Can you work these out from the drawing? Everything is in mm from the part's minimum corner. A direction names the side the tool comes from. Give positions to 0.01 mm unless a question says otherwise; leave off trailing zeros. Order: outer loops, then holes, each group sorted by start corner. A loop starts at its lowest first (then second) coordinate and runs counter-clockwise, first axis right, second up. Notation, with made-up numbers: (76.5, -9.75) -> (86.5, -9.75) arc R15 cw to (86.5, 15.25) -> close; hole circle Ø6 at (53.25, 24.5). An arc over 180 degrees is marked (long way). Answer as CSV lines item,"result". Start each with the question number.
(1) I want a section at B-B (z = 7.5). Please give me the cut outline in (x, y) (3 decimals), plus the area to 4 significant figures.
(2) I need wall thicknesses on L1, parallel to Y at x = 16.5, z = 5.25; L2, parallel to X at y = 7, z = 5.25; L3, parallel to X at y = 5.25, z = 8.5. Which ranges of each line are inside material? Lowest first, please.
(3) On a 3-axis mill with a long thin cutter (end or side, diameter ignored), from which of +Z, -Z, +X, -X, +Y, -Y can I reach the whole of each face in a straight line? I mean the marked faces 1 and 2. Say none if no direction works.
(4) I want a section at C-C (y = 5). Please give me the cut outline in (x, z) (3 decimals), plus the area to 3 significant figures.
(5) I want a section at A-A (x = 29.09). Please give me the cut outline in (y, z) (3 decimals).
(6) Will these pins go through, and if not, where does the flat tip stop? pin 1 Ø6 at (x, y) = (30, 7) entering from +Z (3 decimals); pin 2 Ø7.5 at (x, z) = (16.5, 10) entering from +Y; pin 3 Ø1 at (x, y) = (30.5, 9.5) entering from -Z.
(7) I want a section at D-D (x = 10). Please give me the cut outline in (y, z).
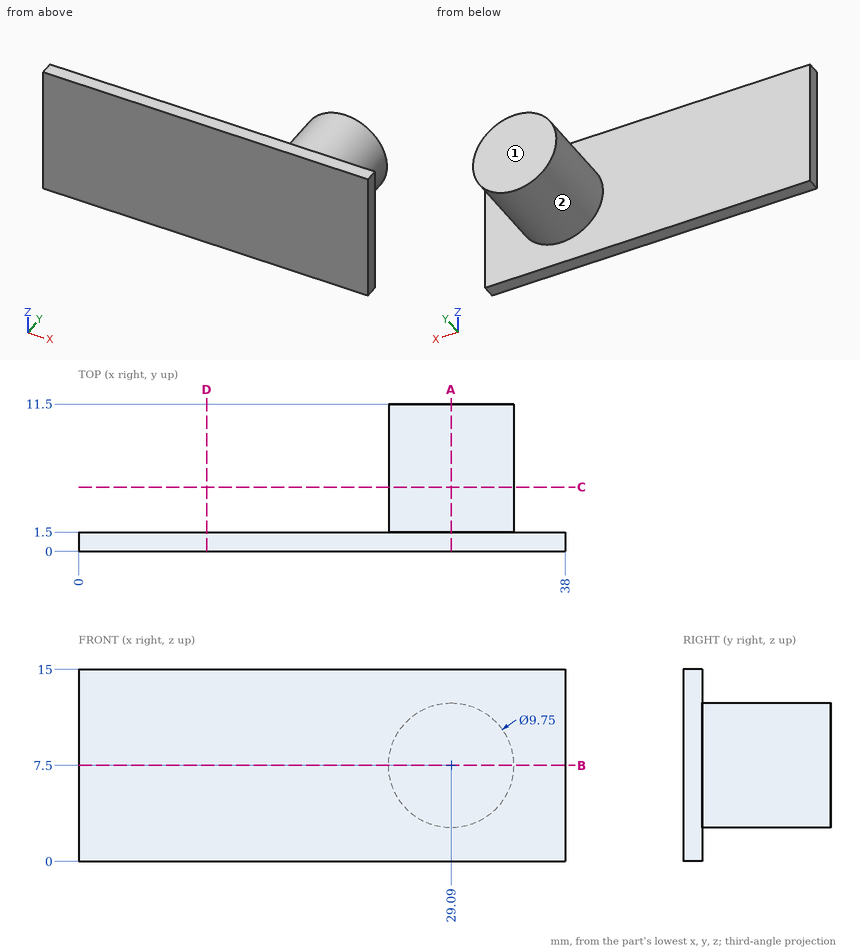
Final values:
1,outline,"(0, 0) -> (38, 0) -> (38, 1.5) -> (33.965, 1.5) -> (33.965, 11.5) -> (24.215, 11.5) -> (24.215, 1.5) -> (0, 1.5) -> close"
1,area,"154.5 mm²"
2,L1,"0 to 1.5"
2,L2,"24.77 to 33.41"
2,L3,"24.32 to 33.86"
3,face 1,"+Z, -Z, +X, -X, +Y"
3,face 2,"+Y"
4,outline,"circle Ø9.75 at (29.09, 7.5)"
4,area,"74.7 mm²"
5,outline,"(0, 0) -> (1.5, 0) -> (1.5, 2.625) -> (11.5, 2.625) -> (11.5, 12.375) -> (1.5, 12.375) -> (1.5, 15) -> (0, 15) -> close"
6,pin 1,"z = 12.375"
6,pin 2,"y = 1.5"
6,pin 3,"z = 2.71"
7,outline,"(0, 0) -> (1.5, 0) -> (1.5, 15) -> (0, 15) -> close"
